Can you work these out from the model? Positions are in its coordinate system, mm. A direction names the side the tool comes from. Coordinates: 2 decimals unless noted, no trailing zeros. Write each loop counter-clockwise with the first axis right and the second up, starting at its lowest first coordinate (ties: lowest second). Pieces come first, ordered by that corner, then holes. Notation, with made-up numbers: (15, -30.5) -> (62, -30.5) arc R24 cw to (62, -12.5) -> close; hole circle Ø11 at (-22, -33.5). An arc over 180 degrees is marked (long way). Answer as CSV lines item,"result". Start each with the question number.
Autodesk Inventor part; units mm, degrees
ref_plane "YZ Plane" through (0, 0, 0) normal (1, 0, 0) x (0, 1, 0)
ref_plane "XZ Plane" through (0, 0, 0) normal (0, 1, 0) x (-1, 0, 0)
ref_plane "XY Plane" through (0, 0, 0) normal (0, 0, 1) x (1, 0, 0)
sketch "Sketch1" plane through (0, 0, 0) normal (0, 1, 0) x (-1, 0, 0)
  circle A0 centre (2.1306, 2.1694) radius 15.5
  line L0 (2.1306, 17.6694) -> (2.1306, 38.1694)
  line L1 (2.1306, -13.3306) -> (2.1306, -33.8306)
  line L2 (2.1306, 38.1694) -> (-57.8694, 38.1694)
  line L3 (2.1306, -33.8306) -> (-57.8694, -33.8306)
  line L4 (-57.8694, -33.8306) -> (-57.8694, 38.1694)
  line L5 (2.1306, 38.1694) -> (34.8074, 38.1694)
  line L6 (34.8074, 38.1694) -> (34.8074, -33.8306)
  line L7 (34.8074, -33.8306) -> (2.1306, -33.8306)
  circle A1 centre (2.1306, 2.1694) radius 15.25
  point P0 (0, 0)
  dimension "d0" = 31
  dimension "d1" = 20.5
  dimension "d2" = 20.5
  dimension "d3" = 60
  dimension "d4" = 30.5
extrude "Extrusion1" add sketch "Sketch1" along normal blind 20 contours A0 L1 L3 L4 L2 L0
ref_plane "Work Plane1" through (-2.1306, 0, 38.1694) normal (0, 0, 1) x (1, 0, 0)
sketch "Sketch2" plane through (-2.1306, 0, 38.1694) normal (0, 0, 1) x (1, 0, 0)
  line L0 (60, 0) -> (60, 20)
  line L1 (60, 10) -> (50, 10)
  circle A0 centre (50, 10) radius 4.1
  point P0 (2.1306, 0)
  dimension "d31" = 8.2
extrude "Extrusion2" cut sketch "Sketch2" against normal blind 192.5
ref_plane "Work Plane2" through (-2.1306, 0, 17.6694) normal (-1, 0, 0) x (0, 0, 1)
sketch "Sketch3" plane through (-2.1306, 0, 17.6694) normal (-1, 0, 0) x (0, 0, 1)
  point P0 (-17.6694, 0)
sketch "Sketch4" plane through (-2.1306, 0, 17.6694) normal (-1, 0, 0) x (0, 0, 1)
  line L0 (20.5, 0) -> (20.5, 20)
  circle A0 centre (14.5, 10) radius 4
  point P0 (-17.6694, 0)
  dimension "d14" = 8
sketch "Sketch5" plane through (-2.1306, 0, 38.1694) normal (0, 0, 1) x (1, 0, 0)
  line L0 (0, 0) -> (0, 20)
  line L1 (60, 0) -> (0, 0)
  line L2 (10, 0) -> (18, 0)
  line L3 (18, 0) -> (18, 20.6661)
  line L4 (18, 20.6661) -> (10, 20.6661)
  line L5 (10, 20.6661) -> (10, 0)
  point P0 (2.1306, 0)
  dimension "d16" = 8
extrude "Extrusion3" cut sketch "Sketch5" against normal blind 12
extrude "Extrusion4" cut sketch "Sketch4" against normal blind 12.5
ref_plane "Work Plane3" through (-2.1306, 0, -33.8306) normal (-1, 0, 0) x (0, 0, 1)
sketch "Sketch6" plane through (-2.1306, 0, -33.8306) normal (-1, 0, 0) x (0, 0, 1)
  line L0 (0, 6) -> (0, 14)
  circle A0 centre (6, 10) radius 4
  point P0 (33.8306, 0)
  dimension "d23" = 8
ref_plane "Work Plane4" through (57.8694, 0, -33.8306) normal (0, 0, -1) x (-1, 0, 0)
sketch "Sketch7" plane through (57.8694, 0, -33.8306) normal (0, 0, -1) x (-1, 0, 0)
  line L0 (60, 0) -> (60, 20)
  line L1 (50, 0) -> (50, 20)
  line L2 (50, 10) -> (50, 20)
  line L3 (0, 0) -> (60, 0)
  line L4 (50, 20) -> (42, 20)
  line L5 (42, 20) -> (42, 0)
  line L6 (42, 0) -> (50, 0)
  line L7 (50, 0) -> (50, 20)
  point P0 (57.8694, 0)
  dimension "d26" = 8
extrude "Extrusion5" cut sketch "Sketch7" against normal blind 12
extrude "Extrusion6" cut sketch "Sketch6" against normal blind 11.75
sketch "Sketch8" plane through (-2.1306, 0, 17.6694) normal (-1, 0, 0) x (0, 0, 1)
  point P0 (-17.6694, 0)
properties part number "BIKE"
Q1. I need wall thicknesses on L1, parallel to X at y = 1.5, z = 29; L2, parallel to Y at x = 2.5, z = -24.5; L3, parallel to Z at x = 12, y = 10.25. Which ranges of each line are inside material? Lowest first, please.
Q2. Imagine slicing it at C-C (y = 10). Write out the boundary of the cut face in (x, z).
Q3. Imagine slicing it at A-A (x = 6). Write out the boundary of the cut face in (y, z), then the cut area to 3 significant figures.
Q4. If we mould it in two halves opening along Z, with no side actions, what happens to faces 5 (the face through (15.869, 10, -28)), 6 (the face through (12, 10, 26.169)), 7 (the face through (13.366, 9.86, 1.829))? For each: released by +Z, released by -Z, zero draft, split by the parting line, or undercut.
Q5. Imagine slicing it at D-D (z = -15). Write out the boundary of the cut face in (x, y), then the cut area to 3 significant figures.
Q6. For pin 1 (4 mm diameter, centred on x = 13, y = 12, fed in from +Z); pin 2 (3.5 mm diameter, centred on y = 11, z = -26.5, fed in from -X); pin 3 (5 mm diameter, centred on x = 47.87, y = 10, fed in from -Z); pin 4 (6.5 mm diameter, centred on x = 11, y = 8, fed in from -Z), each with a flat end and sliding along its axis, tell me the tip position at first contact or that it passes through.
Q7. Imagine slicing it at B-B (z = -25). Write out the boundary of the cut face in (x, y), then the cut area to 3 significant figures.
Q8. Which directions (+Z, -Z, +X, -X, +Y, -Y) give clear straight access to the entire face, cutting with the end or side of a thin tool? Please do faces 1 (the face through (15.869, 10, 32)), 2 (the face through (2.799, 11.201, -24.015)), 3 (the face through (-2.131, 10, 28)), 4 (the face through (12, 10, -21.831)).
Entries:
1,L1,"-2.13 to 7.87, 15.87 to 57.87"
1,L2,"0 to 7.78, 12.22 to 20"
1,L3,"-21.83 to -4.2, 8.54 to 26.17"
2,outline,"(-2.13, -33.83) -> (7.87, -33.83) -> (7.87, -31.83) -> (-2.13, -31.83) -> close; (-2.13, -23.83) -> (7.87, -23.83) -> (7.87, -21.83) -> (15.87, -21.83) -> (15.87, -33.83) -> (43.77, -33.83) -> (43.77, 38.17) -> (15.87, 38.17) -> (15.87, 26.17) -> (7.87, 26.17) -> (7.87, 28.17) -> (-2.13, 28.17) -> (-2.13, 17.67) arc R15.5 cw to (-2.13, -13.33) -> close; (-2.13, 36.17) -> (7.87, 36.17) -> (7.87, 38.17) -> (-2.13, 38.17) -> close; (51.97, -33.83) -> (57.87, -33.83) -> (57.87, 38.17) -> (51.97, 38.17) -> close"
3,outline,"(0, -33.83) -> (20, -33.83) -> (20, -11.03) -> (0, -11.03) -> close; (0, 15.37) -> (20, 15.37) -> (20, 38.17) -> (0, 38.17) -> close; hole circle Ø8 at (10, -27.83); hole circle Ø8 at (10, 32.17)"
3,area,"812 mm2"
4,face 5,"zero draft"
4,face 6,"released by +Z"
4,face 7,"undercut"
5,outline,"(-2.13, 0) -> (57.87, 0) -> (57.87, 20) -> (-2.13, 20) -> close; hole circle Ø8.2 at (47.87, 10)"
5,area,"1,150 mm2"
6,pin 1,"z = 26.17"
6,pin 2,"x = 15.87"
6,pin 3,"through"
6,pin 4,"z = -33.83"
7,outline,"(-2.13, 0) -> (7.87, 0) -> (7.87, 7.17) -> (-2.13, 7.17) -> close; (-2.13, 12.83) -> (7.87, 12.83) -> (7.87, 20) -> (-2.13, 20) -> close; (15.87, 0) -> (57.87, 0) -> (57.87, 20) -> (15.87, 20) -> close; hole circle Ø8.2 at (47.87, 10)"
7,area,"931 mm2"
8,face 1,"+Z, +Y, -Y"
8,face 2,"-X"
8,face 3,"+Z, -Z, -X, +Y, -Y"
8,face 4,"-Z, +Y, -Y"
